```python
from build123d import *

# Parameters (mm, degrees)
F0_R          = 3.81
F1_DEPTH      = 52.3494
F3_DEPTH      = 25.4
F3_DEPTH_BACK = 25.4
F4_DEPTH      = 6.35
F4_DEPTH_BACK = 6.985
F6_DEPTH      = 18.415
F6_DEPTH_BACK = 18.415
F7_R          = 8.89
F8_DEPTH      = 66.62603


with BuildPart() as f1:
    # F0 (on Front) → F1 (new body)
    with BuildSketch(Plane.XZ):
        Circle(F0_R)
    extrude(amount=F1_DEPTH)

    # F2 (on Top) → F3 (cut, two sides)
    with BuildSketch(Plane.XY) as f3_sk:
        with BuildLine():
            Line((0, 0), (-11.43, 0))
            ThreePointArc((-11.43, 0), (-11.0405321945, -2.9583016855), (-9.8986703653, -5.715))
            Line((-9.8986703653, -5.715), (0, 0))
        make_face()
        with BuildLine():
            ThreePointArc((-9.8986703653, -5.715), (0, -11.43), (9.8986703653, -5.715))
            Line((9.8986703653, -5.715), (0, 0))
            Line((0, 0), (-9.8986703653, -5.715))
        make_face()
        with BuildLine():
            ThreePointArc((9.8986703653, -5.715), (11.0405321945, -2.9583016855), (11.43, 0))
            Line((11.43, 0), (0, 0))
            Line((0, 0), (9.8986703653, -5.715))
        make_face()
    extrude(amount=F3_DEPTH, mode=Mode.SUBTRACT)
    extrude(f3_sk.sketch, amount=-F3_DEPTH_BACK, mode=Mode.SUBTRACT)

    # F2 (on Top) → F4 (join, two sides)
    with BuildSketch(Plane.XY) as f4_sk:
        with BuildLine():
            Line((13.1982271537, -7.62), (9.8986703653, -5.715))
            ThreePointArc((9.8986703653, -5.715), (0, -11.43), (-9.8986703653, -5.715))
            Line((-9.8986703653, -5.715), (-13.1982271537, -7.62))
            ThreePointArc((-13.1982271537, -7.62), (0, -15.24), (13.1982271537, -7.62))
        make_face()
    extrude(amount=F4_DEPTH)
    extrude(f4_sk.sketch, amount=-F4_DEPTH_BACK)

    # F5 (on Top) → F6 (join, two sides)
    with BuildSketch(Plane.XY) as f6_sk:
        with BuildLine():
            ThreePointArc((0, -48.5394), (-2.6940768363, -55.0434768363), (3.81, -52.3494))
            ThreePointArc((3.81, -52.3494), (2.6940768363, -49.6553231637), (0, -48.5394))
        make_face()
    extrude(amount=F6_DEPTH)
    extrude(f6_sk.sketch, amount=-F6_DEPTH_BACK)

    # F7 (on Front) → F8 (cut)
    with BuildSketch(Plane.XZ):
        with Locations((0, -18.415)):
            Circle(F7_R)
    extrude(amount=F8_DEPTH, mode=Mode.SUBTRACT)


solid = f1.part
```
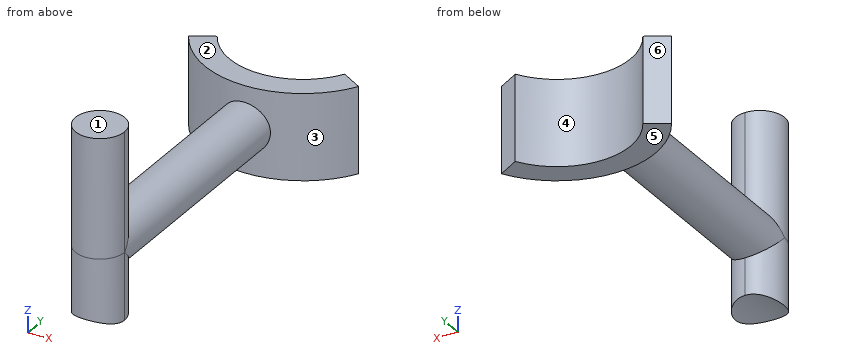
Geometry check sheet. Reference: the model listing, model coordinates, mm. Face numbers are marked on the shaded views. A direction names the side the tool comes from. Coordinates: 2 decimals unless noted, no trailing zeros. Order: outer loops, then holes, each group sorted by start corner. A loop starts at its lowest first (then second) coordinate and runs counter-clockwise, first axis right, second up. Notation, with made-up numbers: (11, -23) - (36, -23) arc R29 ccw to (36, 13) - close; hole circle Ø7 at (77, -14.75). An arc over 180 degrees is marked (long way). Answer as a JSON object with one key per item and string values. Group by question number.
Item 1: Draft check along X on the marked faces 4, 5 and 6. Enter one of: +X half, -X half, draft (parallel to the pull), parting line (faces both ways), or undercut.
Item 2: Sectioned sample at A-A, the plane z = 5.25. Record the cut outline in (x, y) (3 decimals), and give its area (3 significant figures).
Item 3: Scan lines: probe 1 along Z at (x, y) = (-0.25, -38.5); probe 2 along Y at (x, z) = (9.5, 2); probe 3 along Z at (x, y) = (3.5, -44). Record each from-to range of solid material in increasing order.
Item 4: Tool access check on the marked faces 1, 2 and 3. Record the directions out of +Z, -Z, +X, -X, +Y, -Y that give a thin tool (end or side, any length) a straight path to the whole face; none if there is none.
Item 5: Sectioned sample at C-C, the plane z = -8.5. Record the cut outline in (x, y), and give its area (3 significant figures).
Item 6: Sectioned sample at B-B, the plane y = -18.5. Record the cut outline in (x, z), and give its area (3 significant figures).
Item 7: Sectioned sample at D-D, the plane x = -9. Record the cut outline in (y, z) (3 decimals), and give its area (3 significant figures).
Item 8: Depth check by flat-ended pin: pin 1 Ø6 at (x, y) = (-5.5, -40) entering from +Z; pin 2 Ø3 at (y, z) = (-49, -3) entering from -X; pin 3 Ø6 at (x, y) = (-2.5, -24.5) entering from -Z. Enter the tip coordinate at first touch or a pass-through.
Resolved:
{
 "1": {"face 4": "undercut", "face 5": "draft", "face 6": "-X half"},
 "2": {"outline": "(-13.198, -7.62) arc R15.24 ccw to (13.198, -7.62) - (9.899, -5.715) arc R11.43 cw to (-9.899, -5.715) - close; circle Ø7.62 at (0, -52.349)", "area": "152 mm^2"},
 "3": {"probe 1": "-3.8 to 3.8", "probe 2": "-11.92 to -6.36", "probe 3": "-1.51 to 1.51"},
 "4": {"face 1": "+Z, +X, -X, +Y, -Y", "face 2": "+Z, +X, -X, +Y", "face 3": "none"},
 "5": {"outline": "circle Ø7.62 at (0, -52.35)", "area": "45.6 mm^2"},
 "6": {"outline": "circle Ø7.62 at (0, 0)", "area": "45.6 mm^2"},
 "7": {"outline": "(-12.299, -6.985) - (-7.046, -6.985) - (-7.046, 6.35) - (-12.299, 6.35) - close", "area": "70.0 mm^2"},
 "8": {"pin 1": "z = 2.88", "pin 2": "x = -3.5", "pin 3": "z = -3.81"}
}
